```python
from build123d import *

# Parameters (mm, degrees)
SKETCH1_R            = 9
BOSS_EXTRUDE1_DEPTH  = 8.6
SKETCH2_W            = 9.699094827
SKETCH2_H            = 6.5
SKETCH3_R            = 2
CUT_EXTRUDE1_DEPTH   = 9.6
CUT_SWEEP2_PROFILE_R = 0.5
CUT_SWEEP3_PROFILE_R = 0.5


with BuildPart() as part:
    # Sketch1 → Boss-Extrude1 (new body)
    with BuildSketch(Plane(origin=(0, 0, 0), x_dir=(1, 0, 0), z_dir=(0, 1, 0))):
        Circle(SKETCH1_R)
    extrude(amount=BOSS_EXTRUDE1_DEPTH)

    # Sketch2 → Cut-Revolve1 (revolve, cut)
    with BuildSketch(Plane.XY):
        with Locations((-10.849547414, 4.3)):
            Rectangle(SKETCH2_W, SKETCH2_H)
    revolve(axis=Axis((0, 8.6, 0), (0, -1, 0)), mode=Mode.SUBTRACT)

    # Sketch3 → Cut-Extrude1 (cut, through all)
    with BuildSketch(Plane(origin=(0, 8.6, 0), x_dir=(1, 0, 0), z_dir=(0, 1, 0))):
        Circle(SKETCH3_R)
    extrude(amount=-CUT_EXTRUDE1_DEPTH, mode=Mode.SUBTRACT)

    # Cut-Sweep2: sweep along a path in Sketch4
    with BuildLine(Plane(origin=(0, 8.6, 0), x_dir=(1, 0, 0), z_dir=(0, 1, 0))) as cut_sweep2_path:
        CenterArc((0, 0), 4.703999497, 0, 360)
    # Cut-Sweep2 profile (on start of the path) → Cut-Sweep2 (sweep, cut)
    with BuildSketch(Plane(origin=(4.703999497, 8.6, 0), x_dir=(-1, 0, 0), z_dir=(0, 0, -1))):
        Circle(CUT_SWEEP2_PROFILE_R)
    sweep(path=cut_sweep2_path.line, mode=Mode.SUBTRACT)

    # Cut-Sweep3: sweep along a path in Sketch20
    with BuildLine(Plane.XZ) as cut_sweep3_path:
        CenterArc((0, 0), 4.7, 0, 360)
    # Cut-Sweep3 profile (on start of the path) → Cut-Sweep3 (sweep, cut)
    with BuildSketch(Plane(origin=(4.7, 0, 0), x_dir=(1, 0, 0), z_dir=(0, 0, 1))):
        Circle(CUT_SWEEP3_PROFILE_R)
    sweep(path=cut_sweep3_path.line, mode=Mode.SUBTRACT)


solid = part.part
```
The listing builds one solid part. Answer for the finished solid, in the listing's coordinates (mm). A direction names the side the tool comes from. Round coordinates to 2 decimals unless told otherwise and drop trailing zeros. Write each loop counter-clockwise with the first axis right and the second up, starting at its lowest first coordinate (ties: lowest second). Pieces come first, ordered by that corner, then holes. Notation, with made-up numbers: (14, -3) -> (61, -3) arc R14 cw to (61, 17) -> close; hole circle Ø10 at (6.5, -32.75). An arc over 180 degrees is marked (long way). Answer as a JSON object with one key per item and string values. Group by question number.
Q1. Section A-A (x = -7) is taken. Write down the section's boundary in (y, z), plus the area to 3 significant figures.
Q2. Each of these flat-tipped pins is pushed along its axis until it touches: pin 1 Ø3.5 at (x, z) = (0, 0) entering from +Y; pin 2 Ø3 at (x, y) = (-3, 1.5) entering from +Z; pin 3 Ø5.5 at (x, z) = (1.5, 4) entering from -Y; pin 4 Ø1.5 at (x, y) = (4.5, 1) entering from +Z. Where does it stop, or does it pass through?
Q3. Section B-B (z = 7.25) is taken. Write down the section's boundary in (x, y).
Q4. Straight lines are drawn through the part: line 1 along Y through (x, z) = (-6.25, 4.25); line 2 along X through (y, z) = (3.25, 0). For each, find the intervals that lie inside material, in ascending order.
Q5. Section C-C (y = 5) is taken. Write down the section's boundary in (x, z).
Q6. Which of the six approach directions +Z, -Z, +X, -X, +Y, -Y give full straight-line access (tool end or side, diameter ignored) to faces 1 (the face through (-2, 7.55, 6)), 2 (the face through (1, 8.6, 2))?
Q7. Determine the mould class of faces 3 (the face through (0, 4, 2)), 4 (the face through (4, 8.6, 4)), 5 (the face through (0.78, 4.35, -5.95)) for opening direction Z: pulls with the +Z half, pulls with the -Z half, needs draft (parallel to the pull), parting line crosses it, or undercut.
Check values:
{
 "1": {"outline": "(0, -5.66) -> (1.05, -5.66) -> (1.05, 5.66) -> (0, 5.66) -> close; (7.55, -5.66) -> (8.6, -5.66) -> (8.6, 5.66) -> (7.55, 5.66) -> close", "area": "23.8 mm^2"},
 "2": {"pin 1": "through", "pin 2": "z = 8.86", "pin 3": "y = 0", "pin 4": "z = 8.18"},
 "3": {"outline": "(-5.33, 0) -> (5.33, 0) -> (5.33, 1.05) -> (-5.33, 1.05) -> close; (-5.33, 7.55) -> (5.33, 7.55) -> (5.33, 8.6) -> (-5.33, 8.6) -> close"},
 "4": {"line 1": "0 to 1.05, 7.55 to 8.6", "line 2": "-6 to -2, 2 to 6"},
 "5": {"outline": "circle Ø12 at (0, 0); hole circle Ø4 at (0, 0)"},
 "6": {"face 1": "none", "face 2": "+Z, -Z, +X, -X, +Y"},
 "7": {"face 3": "undercut", "face 4": "needs draft", "face 5": "parting line crosses it"}
}
